Autodesk Inventor part; units mm, degrees
ref_plane "YZ Plane" through (0, 0, 0) normal (1, 0, 0) x (0, 1, 0)
ref_plane "XZ Plane" through (0, 0, 0) normal (0, 1, 0) x (-1, 0, 0)
ref_plane "XY Plane" through (0, 0, 0) normal (0, 0, 1) x (1, 0, 0)
sketch "Esquisse1" plane through (0, 0, 0) normal (0, 0, 1) x (1, 0, 0)
  circle A0 centre (0, 0) radius 1.2
  circle A1 centre (0, 0) radius 3
  circle A2 centre (0, 11.8) radius 2
  circle A3 centre (0, 11.8) radius 2.75
  circle A4 centre (0, -11.8) radius 2.75
  circle A5 centre (0, -11.8) radius 2
  circle A6 centre (0, 11.8) radius 1.5
  circle A7 centre (0, -11.8) radius 1.5
  arc A8 (-1.4212, 14.1543) -> (-1.4212, -14.1543) centre (0, 0) ccw
  arc A9 (1.4212, -14.1543) -> (1.4212, 14.1543) centre (0, 0) ccw
  circle A10 centre (0, 0) radius 14.75
  dimension "d1" = 2.4
  dimension "d2" = 6
  dimension "d3" = 4
  dimension "d4" = 11.8
  dimension "d5" = 5.5
  dimension "d8" = 360
  dimension "d12" = 3
  dimension "d15" = 360
  dimension "d95" = 29.5
extrude "Extrusion10" add sketch "Esquisse1" along normal blind 3 contours A3 A9 A4 A8 | A10
extrude "Extrusion11" add sketch "Esquisse1" along normal blind 6 contours A1
extrude "Extrusion12" add sketch "Esquisse1" along normal blind 0.5 contours A2 | A5
extrude "Extrusion13" add sketch "Esquisse1" along normal blind 1.5 contours A3 | A4
sketch "Esquisse3" plane through (0, 0, 3) normal (0, 0, 1) x (1, 0, 0)
  circle A0 centre (0, 0) radius 1.2
  line L0 (0, 0) -> (-7.6468, 0)
  circle A1 centre (0, 0) radius 3
  line L1 (0, 0) -> (4.4865, 0)
  line L2 (0, 16.0443) -> (0, -15.4592)
  line L3 (0, 0) -> (-3.7622, -10.3366)
  line L4 (0, 0) -> (3.7622, -10.3366)
  line L5 (0, 0) -> (3.7622, 10.3366)
  line L6 (0, 0) -> (-3.7622, 10.3366)
  arc A2 (3.7622, -10.3366) -> (3.7622, 10.3366) centre (0, 0) ccw
  arc A3 (-3.7622, 10.3366) -> (-3.7622, -10.3366) centre (0, 0) ccw
  arc A4 (2.0521, -5.6382) -> (2.0521, 5.6382) centre (0, 0) ccw
  arc A5 (-2.0521, 5.6382) -> (-2.0521, -5.6382) centre (0, 0) ccw
  dimension "d75" = 360
  dimension "d71" = 20
  dimension "d72" = 40
extrude "Extrusion15" cut sketch "Esquisse3" against normal through all contours L5 A2 L4 A4 | A5 L3 A3 L6
fillet "Congé1" radius 2 8 edges at (3.7622, -10.3366, 1.5) (-3.7622, -10.3366, 1.5) (-3.7622, 10.3366, 1.5) (3.7622, 10.3366, 1.5) (-2.0521, -5.6382, 1.5) (-2.0521, 5.6382, 1.5) (2.0521, -5.6382, 1.5) (2.0521, 5.6382, 1.5)
chamfer "Chanfrein1" distance 0.5 angle 45 1 edges at (-3, 0, 3)
sketch "Esquisse5" plane through (0, 0, 3) normal (0, 0, 1) x (1, 0, 0)
  circle A0 centre (0, -11.8) radius 1.5
  arc A1 (2.1004, -14.5997) -> (-2.1004, -14.5997) centre (0, -11.8) ccw
  circle A2 centre (0, 11.8) radius 2.75
  arc A3 (-2.1004, 14.5997) -> (2.1004, 14.5997) centre (0, 11.8) ccw
  circle A4 centre (0, -11.8) radius 2.75
  circle A5 centre (0, 11.8) radius 2.75
  circle A6 centre (0, 0) radius 1.2
  circle A7 centre (0, 0) radius 14.75
  arc A8 (-2.1004, -14.5997) -> (2.1004, -14.5997) centre (0, 0) ccw
  arc A9 (2.1004, 14.5997) -> (-2.1004, 14.5997) centre (0, 0) ccw
  circle A10 centre (0, -11.8) radius 2.75
  dimension "d96" = 7
  dimension "d97" = 7
extrude "Extrusion18" add sketch "Esquisse5" along normal blind 1.5 contours A7 A1 | A7 A3
sketch "Esquisse6" plane through (0, 0, 4.5) normal (0, 0, 1) x (1, 0, 0)
  line L0 (-1.5, -15.5653) -> (1.5, -15.5653)
  line L1 (1.5, -15.5653) -> (1.5, -13.8468)
  line L2 (1.5, -13.8468) -> (-1.5, -13.8468)
  line L3 (-1.5, -13.8468) -> (-1.5, -15.5653)
  line L4 (0, 0) -> (0, -17.5217)
  dimension "d104" = 3
  dimension "d105" = 1.5
extrude "Extrusion19" cut sketch "Esquisse6" against normal blind 3
pattern_circular "Réseau circulaire3" count 2 over 360 about axis through (0, 0, 0) along (0, 0, 1) of "Extrusion19"
fillet "Congé3" radius 0.5 2 edges at (0, -8.3, 3) (0, 8.3, 3)
equation "\"d105\" = 0.5 * d104"
properties part number "magnet_holder-july21"
The model under review builds one solid part; all positions refer to its coordinate system, in mm. A direction names the side the tool comes from. Give positions to 0.01 mm unless a question says otherwise; leave off trailing zeros. Loops run counter-clockwise (first coordinate to the right, second up) from the corner with the lowest first, then second, coordinate; pieces in that order, holes last. Notation, with made-up numbers: (21, 85) -> (80, 85) arc R9 cw to (80, 98) -> close; hole circle Ø8 at (-39, 11.25). An arc over 180 degrees is marked (long way). Put each result on its own line as item: value. Start each with the question number.
1. We need section D-D on x = 0.5. State how many separate pieces and enclosed holes the cut face has, then the cut area to 3 significant figures.
2. Mouldability with a two-part tool opening along Y and no side actions: class faces 1 (the face through (-1, -9, 4.5)), 2 (the face through (-1.92, -14.624, 1.719)), 3 (the face through (2.63, 5.97, 1.48)), 4 (the face through (-2.823, -7.756, 1.521)) as released by +Y, released by -Y, zero draft, split by the parting line, or undercut.
3. We need section A-A on y = 11.8. State the section outline as (x, z) points, then the cut area to 3 significant figures.
4. We need section B-B on z = 4. State the section outline as (x, y) points, then the cut area to 3 significant figures.
5. Clearance check with flat-ended pins moving along their axes: P1, Ø5, axis at x = -6, y = 3, coming from the -Z side; P2, Ø7, axis at x = -1, y = -11.5, coming from the +Z side; P3, Ø1.5, axis at y = 9.5, z = 3.5, coming from the -X side; P4, Ø0.5, axis at y = -14.5, z = 3.5, coming from the -X side. State where each tip first meets the part, or that it passes through.
6. Wall thickness on probe 1 along Y at (x, z) = (0, 3.5); probe 2 along Y at (x, z) = (0, 0.35); probe 3 along Y at (x, z) = (0, 2.7): over which ranges is each line inside the solid? List them lowest first.
7. For faces 5 (the face through (11, 0, 2)), 6 (the face through (-0.1, -8.3, 4)), 7 (the face through (1, 9, 4.5)), list the 3-axis set-ups (+Z, -Z, +X, -X, +Y, -Y) from which the entire face can be reached by the end or side of a thin tool; tool diameter is ignored.
8. We need section C-C on y = 0. State the section outline as (x, z) points, then the cut area to 3 significant figures.
Determined:
1. separate pieces: 4
1. enclosed holes: 0
1. area: 68.2 mm^2
2. face 1: zero draft
2. face 2: split by the parting line
2. face 3: undercut
2. face 4: undercut
3. outline: (-8.85, 0) -> (-1.5, 0) -> (-1.5, 0.5) -> (-2, 0.5) -> (-2, 1.5) -> (-2.75, 1.5) -> (-2.75, 4.5) -> (-3.5, 4.5) -> (-3.5, 3.5) arc R0.5 cw to (-4, 3) -> (-8.85, 3) -> close; (1.5, 0) -> (8.85, 0) -> (8.85, 3) -> (4, 3) arc R0.5 cw to (3.5, 3.5) -> (3.5, 4.5) -> (2.75, 4.5) -> (2.75, 1.5) -> (2, 1.5) -> (2, 0.5) -> (1.5, 0.5) -> close
3. area: 41.7 mm^2
4. outline: circle Ø6 at (0, 0); (-2.1, -14.6) arc R14.75 ccw to (-1.5, -14.67) -> (-1.5, -14.1) arc R2.75 cw (long way) to (1.5, -14.1) -> (1.5, -14.67) arc R14.75 ccw to (2.1, -14.6) arc R3.5 ccw (long way) to start; (-2.1, 14.6) arc R3.5 ccw (long way) to (2.1, 14.6) arc R14.75 ccw to (1.5, 14.67) -> (1.5, 14.1) arc R2.75 cw (long way) to (-1.5, 14.1) -> (-1.5, 14.67) arc R14.75 ccw to start; hole circle Ø2.4 at (0, 0)
4. area: 48.1 mm^2
5. P1: z = 0
5. P2: z = 4.5
5. P3: x = -11.73
5. P4: x = -2.5
6. probe 1: -9.05 to -8.3, -3 to -1.2, 1.2 to 3, 8.3 to 9.05
6. probe 2: -14.75 to -13.3, -10.3 to -1.2, 1.2 to 10.3, 13.3 to 14.75
6. probe 3: -9.05 to -1.2, 1.2 to 9.05
7. face 5: +Z, -Z
7. face 6: +Z
7. face 7: +Z, +X, -X, +Y
8. outline: (-14.75, 0) -> (-11, 0) -> (-11, 3) -> (-14.75, 3) -> close; (-6, 0) -> (-1.2, 0) -> (-1.2, 6) -> (-3, 6) -> (-3, 3.5) -> (-3.5, 3) -> (-6, 3) -> close; (1.2, 0) -> (6, 0) -> (6, 3) -> (3.5, 3) -> (3, 3.5) -> (3, 6) -> (1.2, 6) -> close; (11, 0) -> (14.75, 0) -> (14.75, 3) -> (11, 3) -> close
8. area: 62.4 mm^2
